```python
from build123d import *

# Parameters (mm, degrees)
F1_DEPTH = 20
F3_D     = 3.2
F4_R     = 3
F5_R     = 2


with BuildPart() as f1:
    # F0 (on Front) → F1 (new body)
    with BuildSketch(Plane.XZ):
        Polygon((-24.0542695144, 1.0263364321), (-24.0542695144, -16.9736635679), (-22.0542695144, -16.9736635679), (-22.0542695144, -0.9736635679), (-6.0542695144, -0.9736635679), (-6.0542695144, 1.0263364321), align=None)
    extrude(amount=F1_DEPTH)

    # F3 (through all)
    with Locations(Plane.XY.offset(1.0263364321)):
        with Locations((-14.0542695144, -10)):
            Hole(F3_D / 2)

    # F4
    f4_edges = [f1.edges().sort_by_distance(p)[0] for p in [
        (-24.05427, -10, 1.026336),
    ]]
    fillet(f4_edges, radius=F4_R)

    # F5
    f5_edges = [f1.edges().sort_by_distance(p)[0] for p in [
        (-22.05427, -10, -0.973664),
    ]]
    fillet(f5_edges, radius=F5_R)


solid = f1.part
```
Part model, mm, in its own coordinate system. A direction names the side the tool comes from. Round coordinates to 2 decimals unless told otherwise and drop trailing zeros. Order: outer loops, then holes, each group sorted by start corner. A loop starts at its lowest first (then second) coordinate and runs counter-clockwise, first axis right, second up. Notation, with made-up numbers: M -18.75,-15 L 10.25,-15 A12 cw 10.25,-10 Z; hole C 63.5,-25 d5. An arc over 180 degrees is marked long. Put each result on its own line as item: value. Start each with the question number.
1. Slice it at A-A on y = -10. List the corners of the cut face in (x, z), then the cut area to 3 significant figures.
2. Tool access for faces 4 (the face through (-12, -10, -0.974)), 5 (the face through (-22.4, 0, -3.9)): list every direction of +Z, -Z, +X, -X, +Y, -Y with a clear straight run to the whole face (end or side of a thin tool).
3. Slice it at B-B on x = -13.75. List the corners of the cut face in (y, z).
4. Two-plate mould, pull along X, no slides. Class faces 1 (the face through (-12.78, -10.97, 0.01)), 2 (the face through (-24.054, -10, -9)), 3 (the face through (-22.054, -10, -10)): +X half, -X half, draft (parallel to the pull), parting line (faces both ways), or undercut.
5. Drill centre lines: probe 1 along Z at (x, y) = (-19.25, -15.75); probe 2 along X at (y, z) = (-18, -10.25); probe 3 along Z at (x, y) = (-21.25, -11.5). Where is each one in solid material? Low to high. Write a range as [from, to].
6. Slice it at C-C on y = -14.5. List the corners of the cut face in (x, z), then the cut area to 3 significant figures.
7. Slice it at D-D on z = -0.5. List the corners of the cut face in (x, y), then the cut area to 3 significant figures.
8. Drop flat-ended pins along their axis: pin 1 (7 mm diameter, centred on x = -10, y = -15, fed in from -Z); pin 2 (8 mm diameter, centred on x = -18.5, z = -1, fed in from +Y). Give the stop position or say it passes through.
Findings:
1. outline: M -24.05,-16.97 L -22.05,-16.97 L -22.05,-2.97 A2 cw -20.05,-0.97 L -15.65,-0.97 L -15.65,1.03 L -21.05,1.03 A3 ccw -24.05,-1.97 Z; M -12.45,-0.97 L -6.05,-0.97 L -6.05,1.03 L -12.45,1.03 Z
1. area: 60.5 mm2
2. face 4: -Z, +X, +Y, -Y
2. face 5: +Z, -Z, +X, -X, +Y
3. outline: M -20,-0.97 L -11.57,-0.97 L -11.57,1.03 L -20,1.03 Z; M -8.43,-0.97 L 0,-0.97 L 0,1.03 L -8.43,1.03 Z
4. face 1: undercut
4. face 2: -X half
4. face 3: +X half
5. probe 1: [-0.97, 1.03]
5. probe 2: [-24.05, -22.05]
5. probe 3: [-1.37, 1.02]
6. outline: M -24.05,-16.97 L -22.05,-16.97 L -22.05,-2.97 A2 cw -20.05,-0.97 L -6.05,-0.97 L -6.05,1.03 L -21.05,1.03 A3 ccw -24.05,-1.97 Z
6. area: 66.9 mm2
7. outline: M -23.67,-20 L -6.05,-20 L -6.05,0 L -23.67,0 Z; hole C -14.05,-10 d3.2
7. area: 344 mm2
8. pin 1: z = -0.97
8. pin 2: y = 0
